Part model, mm, in its own coordinate system. A direction names the side the tool comes from. Give positions to 0.01 mm unless a question says otherwise; leave off trailing zeros. Order: outer loops, then holes, each group sorted by start corner. A loop starts at its lowest first (then second) coordinate and runs counter-clockwise, first axis right, second up. Notation, with made-up numbers: M -2.75,-16 L 23.25,-16 A19 cw 23.25,-8 Z; hole C -19,-17 d7. An arc over 180 degrees is marked long. Answer as a JSON object with one key per item and string values.
from build123d import *

# Parameters (mm, degrees)
SKETCH1_R                 = 23
SKETCH1_R_2               = 18
BOSS_EXTRUDE1_DEPTH       = 11
BOSS_EXTRUDE2_START       = 3
SKETCH1_13_R              = 23
SKETCH1_13_R_2            = 18
SKETCH1_13_R_3            = 3
SKETCH1_13_R_4            = 5.25
BOSS_EXTRUDE2_DEPTH       = 3
BOSS_EXTRUDE4_START       = 3
BOSS_EXTRUDE4_OUTLINE_R   = 23
BOSS_EXTRUDE4_OUTLINE_R_2 = 3
BOSS_EXTRUDE4_OUTLINE_R_3 = 5.25
BOSS_EXTRUDE4_DEPTH       = 3
BOSS_EXTRUDE5_START       = 60
SKETCH1_17_R              = 23
SKETCH1_17_R_2            = 18
BOSS_EXTRUDE5_DEPTH       = 60
SKETCH2_R                 = 1.5
CUT_EXTRUDE1_DEPTH        = 5
BOSS_EXTRUDE6_START       = 3
SKETCH1_20_R              = 3
SKETCH1_20_R_2            = 1.5
BOSS_EXTRUDE6_DEPTH       = 3
SKETCH1_21_R              = 23
SKETCH1_21_R_2            = 18
CUT_EXTRUDE4_DEPTH        = 23
SKETCH2_2_R               = 1.5
CUT_EXTRUDE5_DEPTH        = 9
BOSS_EXTRUDE7_START       = -5
SKETCH3_R                 = 30
SKETCH3_R_2               = 23
BOSS_EXTRUDE7_DEPTH       = 5
FILLET1_R                 = 10


# Read off the part's stored shape, not the designer's step: Boss-Extrude4
with BuildPart() as part:
    # Sketch1 → Boss-Extrude1 (new body)
    with BuildSketch(Plane(origin=(0, 0, 0), x_dir=(0, 0, -1), z_dir=(1, 0, 0))):
        Circle(SKETCH1_R)
        Circle(SKETCH1_R_2, mode=Mode.SUBTRACT)
    extrude(amount=-BOSS_EXTRUDE1_DEPTH)

    # Sketch1<13> → Boss-Extrude2 (add)
    # profile 1 of 2: a face of its own
    with BuildSketch(Plane(origin=(0, 0, 0), x_dir=(0, 0, -1), z_dir=(1, 0, 0)).offset(BOSS_EXTRUDE2_START)):
        Circle(SKETCH1_13_R)
        Circle(SKETCH1_13_R_2, mode=Mode.SUBTRACT)
    # profile 2 of 2: a face of its own
    with BuildSketch(Plane(origin=(0, 0, 0), x_dir=(0, 0, -1), z_dir=(1, 0, 0)).offset(BOSS_EXTRUDE2_START)):
        Circle(SKETCH1_13_R_2)
        with Locations((-8.5, 0)):
            Circle(SKETCH1_13_R_3, mode=Mode.SUBTRACT)
        with Locations((8.5, 0)):
            Circle(SKETCH1_13_R_3, mode=Mode.SUBTRACT)
        Circle(SKETCH1_13_R_4, mode=Mode.SUBTRACT)
        with Locations((0, -8.5)):
            Circle(SKETCH1_13_R_3, mode=Mode.SUBTRACT)
        with Locations((0, 8.5)):
            Circle(SKETCH1_13_R_3, mode=Mode.SUBTRACT)
    extrude(amount=-BOSS_EXTRUDE2_DEPTH)

    # Boss-Extrude4 outline → Boss-Extrude4 (add)
    with BuildSketch(Plane(origin=(0, 0, 0), x_dir=(0, 0, -1), z_dir=(1, 0, 0)).offset(BOSS_EXTRUDE4_START)):
        Circle(BOSS_EXTRUDE4_OUTLINE_R)
        with Locations((0, -8.5)):
            Circle(BOSS_EXTRUDE4_OUTLINE_R_2, mode=Mode.SUBTRACT)
        with Locations((-8.5, 0)):
            Circle(BOSS_EXTRUDE4_OUTLINE_R_2, mode=Mode.SUBTRACT)
        Circle(BOSS_EXTRUDE4_OUTLINE_R_3, mode=Mode.SUBTRACT)
        with Locations((8.5, 0)):
            Circle(BOSS_EXTRUDE4_OUTLINE_R_2, mode=Mode.SUBTRACT)
        with Locations((0, 8.5)):
            Circle(BOSS_EXTRUDE4_OUTLINE_R_2, mode=Mode.SUBTRACT)
    extrude(amount=BOSS_EXTRUDE4_DEPTH)

    # Sketch1<17> → Boss-Extrude5 (add)
    with BuildSketch(Plane(origin=(0, 0, 0), x_dir=(0, 0, -1), z_dir=(1, 0, 0)).offset(BOSS_EXTRUDE5_START)):
        Circle(SKETCH1_17_R)
        Circle(SKETCH1_17_R_2, mode=Mode.SUBTRACT)
    extrude(amount=-BOSS_EXTRUDE5_DEPTH)

    # Sketch2 → Cut-Extrude1 (cut)
    with BuildSketch(Plane(origin=(60, 0, 0), x_dir=(0, 0, -1), z_dir=(1, 0, 0))):
        with Locations((0, 20.5)):
            Circle(SKETCH2_R)
        with Locations((20.5, 0)):
            Circle(SKETCH2_R)
        with Locations((0, -20.5)):
            Circle(SKETCH2_R)
        with Locations((-20.5, 0)):
            Circle(SKETCH2_R)
    extrude(amount=-CUT_EXTRUDE1_DEPTH, mode=Mode.SUBTRACT)

    # Sketch1<20> → Boss-Extrude6 (add)
    # profile 1 of 4: a face of its own
    with BuildSketch(Plane(origin=(0, 0, 0), x_dir=(0, 0, -1), z_dir=(1, 0, 0)).offset(BOSS_EXTRUDE6_START)):
        with Locations((0, 8.5)):
            Circle(SKETCH1_20_R)
        with Locations((0, 8.5)):
            Circle(SKETCH1_20_R_2, mode=Mode.SUBTRACT)
    # profile 2 of 4: a face of its own
    with BuildSketch(Plane(origin=(0, 0, 0), x_dir=(0, 0, -1), z_dir=(1, 0, 0)).offset(BOSS_EXTRUDE6_START)):
        with Locations((-8.5, 0)):
            Circle(SKETCH1_20_R)
        with Locations((-8.5, 0)):
            Circle(SKETCH1_20_R_2, mode=Mode.SUBTRACT)
    # profile 3 of 4: a face of its own
    with BuildSketch(Plane(origin=(0, 0, 0), x_dir=(0, 0, -1), z_dir=(1, 0, 0)).offset(BOSS_EXTRUDE6_START)):
        with Locations((0, -8.5)):
            Circle(SKETCH1_20_R)
        with Locations((0, -8.5)):
            Circle(SKETCH1_20_R_2, mode=Mode.SUBTRACT)
    # profile 4 of 4: a face of its own
    with BuildSketch(Plane(origin=(0, 0, 0), x_dir=(0, 0, -1), z_dir=(1, 0, 0)).offset(BOSS_EXTRUDE6_START)):
        with Locations((8.5, 0)):
            Circle(SKETCH1_20_R)
        with Locations((8.5, 0)):
            Circle(SKETCH1_20_R_2, mode=Mode.SUBTRACT)
    extrude(amount=BOSS_EXTRUDE6_DEPTH)

    # Sketch1<21> → Cut-Extrude4 (cut)
    with BuildSketch(Plane(origin=(0, 0, 0), x_dir=(0, 0, -1), z_dir=(1, 0, 0))):
        Circle(SKETCH1_21_R)
        Circle(SKETCH1_21_R_2, mode=Mode.SUBTRACT)
    extrude(amount=-CUT_EXTRUDE4_DEPTH, mode=Mode.SUBTRACT)

    # Sketch2<2> → Cut-Extrude5 (cut)
    with BuildSketch(Plane(origin=(60, 0, 0), x_dir=(0, 0, -1), z_dir=(1, 0, 0))):
        with Locations((0, 20.5)):
            Circle(SKETCH2_2_R)
        with Locations((20.5, 0)):
            Circle(SKETCH2_2_R)
        with Locations((0, -20.5)):
            Circle(SKETCH2_2_R)
        with Locations((-20.5, 0)):
            Circle(SKETCH2_2_R)
    extrude(amount=-CUT_EXTRUDE5_DEPTH, mode=Mode.SUBTRACT)

    # Sketch3 → Boss-Extrude7 (add)
    with BuildSketch(Plane.ZY.offset(BOSS_EXTRUDE7_START)):
        Circle(SKETCH3_R)
        with Locations(Location((0, 0, 0), (0, 0, 180))):
            Circle(SKETCH3_R_2, mode=Mode.SUBTRACT)
    extrude(amount=BOSS_EXTRUDE7_DEPTH)

    # Fillet1
    # the kernel refuses this fillet: 10 mm, written as the material it adds along each edge
    with BuildSketch(Plane(origin=(5, 0, 0), x_dir=(0, 0, -1), z_dir=(0, 1, 0))) as fillet1_piece_1:
        with BuildLine():
            CenterArc((33, -9.539392014), FILLET1_R, 107.457603124, 72.542396876)
            Line((30, 0), (29.94, 0.19078784))
            ThreePointArc((29.94, 0.19078784), (26.5, 0.2), (23, 0.2))
            Line((23, 0.2), (22.8, 0))
            Line((22.8, 0), (22.8, -9.539392014))
            Line((22.8, -9.539392014), (23, -9.539392014))
        make_face()
    revolve(axis=Axis((5, 0, 0), (-1, 0, 0)))


solid = part.part
1. Probe line 1 along Y through (x, z) = (58, 0); line 2 along Z through (x, y) = (56.5, -0.5); line 3 along X through (y, z) = (4, 11.5). List the from-to ranges inside material, lowest first.
Worked answers:
{"line 1": "y = -23 to -22, -19 to -18, 18 to 19, 22 to 23", "line 2": "z = -22.99 to -21.91, -19.09 to -17.99, 17.99 to 19.09, 21.91 to 22.99", "line 3": "x = 0 to 6"}
2. Which spindle directions (+Z, -Z, +X, -X, +Y, -Y) get a long thin tool onto all of the face, cutting with end or side? Do faces 4 (the flat face through (51, 0, 21)), 5 (the cylindrical face through (4, 0, 10)), 6 (the flat face through (3, -1, 10)). Say none if no direction does.
Worked answers:
{"face 4": "+X", "face 5": "+X, -X", "face 6": "-X"}
3. Two-plate mould, pull along Y, no slides. Class faces 1 (the cylindrical face through (56, -19, 0)), 2 (the flat face through (0, -6, 6)), 3 (the cylindrical face through (37.588, 22.804, 2.994)): +Y half, -Y half, draft (parallel to the pull), parting line (faces both ways), or undercut.
Worked answers:
{"face 1": "undercut", "face 2": "draft", "face 3": "parting line"}
4. Cut at A-A on z = 0. State how many separate pieces and enclosed holes the cut face has, plus the area to 3 significant figures.
Worked answers:
{"separate pieces": "4", "enclosed holes": "0", "area": "751 mm^2"}
5. Pin check, flat tips, straight feed: P1, Ø10, axis at x = 30.5, z = 19, coming from the -Y side; P2, Ø2, axis at x = 40, y = 0.5, coming from the -Z side; P3, Ø1.5, axis at x = 50.5, z = -14, coming from the +Y side; P4, Ø2.5, axis at y = 8.5, z = 0, coming from the +X side. Stop position of each tip, or through.
Worked answers:
{"P1": "stops at y = -18.25", "P2": "stops at z = -23", "P3": "stops at y = 18.8", "P4": "passes through"}
6. Cut at B-B on x = 49. Give the cut face in (y, z), plus the area to 3 significant figures.
Worked answers:
{"outline": "C 0,0 d46; hole C 0,0 d36", "area": "644 mm^2"}
